The model under review builds one solid part; all positions refer to its coordinate system, in mm. A direction names the side the tool comes from. Coordinates: 2 decimals unless noted, no trailing zeros. Order: outer loops, then holes, each group sorted by start corner. A loop starts at its lowest first (then second) coordinate and runs counter-clockwise, first axis right, second up. Notation, with made-up numbers: (36, 5.5) -> (40, 5.5) arc R23 ccw to (40, 28.5) -> close; hole circle Ø5 at (18.5, 70). An arc over 180 degrees is marked (long way). Use one line per item in the form item = value.
from build123d import *

# Parameters (mm, degrees)
ESQUISSE1_W      = 112
ESQUISSE1_H      = 112
ESQUISSE1_R      = 1.5
EXTRUSION1_DEPTH = 3
ESQUISSE2_W      = 50.8
ESQUISSE2_H      = 25.4
EXTRUSION2_DEPTH = 10
CONG_1_R         = 2
ESQUISSE3_W      = 10
ESQUISSE3_H      = 10
EXTRUSION3_DEPTH = 10
ESQUISSE4_W      = 30
ESQUISSE4_H      = 10
EXTRUSION4_DEPTH = 25
ESQUISSE6_W      = 25
ESQUISSE6_H      = 5
EXTRUSION6_DEPTH = 10


with BuildPart() as part:
    # Esquisse1 → Extrusion1 (new body)
    with BuildSketch(Plane(origin=(0, 0, 0), x_dir=(1, 0, 0), z_dir=(0, 1, 0))):
        with Locations((56, 56)):
            Rectangle(ESQUISSE1_W, ESQUISSE1_H)
        with Locations((3.55, 108.45)):
            Circle(ESQUISSE1_R, mode=Mode.SUBTRACT)
        with Locations((108.45, 108.45)):
            Circle(ESQUISSE1_R, mode=Mode.SUBTRACT)
        with Locations((108.45, 3.55)):
            Circle(ESQUISSE1_R, mode=Mode.SUBTRACT)
        with Locations((3.55, 3.55)):
            Circle(ESQUISSE1_R, mode=Mode.SUBTRACT)
    extrude(amount=EXTRUSION1_DEPTH)

    # Esquisse2 → Extrusion2 (add)
    with BuildSketch(Plane(origin=(0, 3, 0), x_dir=(1, 0, 0), z_dir=(0, 1, 0))):
        with Locations((76.797974596, 22.38755788)):
            Rectangle(ESQUISSE2_W, ESQUISSE2_H)
    extrude(amount=EXTRUSION2_DEPTH)

    # Congé1
    cong_1_edges = [part.edges().sort_by_distance(p)[0] for p in [
        (51.397974596, 13, -22.38755788),
        (76.797974596, 13, -9.68755788),
        (102.197974596, 13, -22.38755788),
        (76.797974596, 13, -35.08755788),
    ]]
    fillet(cong_1_edges, radius=CONG_1_R)

    # Esquisse3 → Extrusion3 (add)
    with BuildSketch(Plane(origin=(0, 3, 0), x_dir=(1, 0, 0), z_dir=(0, 1, 0))):
        with Locations((110.289997157, 97.226447648)):
            Rectangle(ESQUISSE3_W, ESQUISSE3_H)
        with Locations((110.289997157, 67.226447648)):
            Rectangle(ESQUISSE3_W, ESQUISSE3_H)
        with Locations((110.289997157, 52.226447648)):
            Rectangle(ESQUISSE3_W, ESQUISSE3_H)
        with Locations((110.289997157, 82.226447648)):
            Rectangle(ESQUISSE3_W, ESQUISSE3_H)
    extrude(amount=EXTRUSION3_DEPTH)

    # Esquisse4 → Extrusion4 (add)
    with BuildSketch(Plane(origin=(0, 3, 0), x_dir=(1, 0, 0), z_dir=(0, 1, 0))):
        with Locations((61.461032567, 56.630717004)):
            Rectangle(ESQUISSE4_W, ESQUISSE4_H)
        with Locations((61.461032567, 70.501921666)):
            Rectangle(ESQUISSE4_W, ESQUISSE4_H)
        with Locations((31.569885157, 19.889690111)):
            Rectangle(ESQUISSE4_W, ESQUISSE4_H)
        with Locations((61.461032567, 87.97905365)):
            Rectangle(ESQUISSE4_W, ESQUISSE4_H)
    extrude(amount=EXTRUSION4_DEPTH)

    # Esquisse6 → Extrusion6 (add)
    with BuildSketch(Plane(origin=(0, 3, 0), x_dir=(1, 0, 0), z_dir=(0, 1, 0))):
        with Locations((23.111824989, 78.410936793)):
            Rectangle(ESQUISSE6_W, ESQUISSE6_H)
        with Locations((23.111824989, 57.971644922)):
            Rectangle(ESQUISSE6_W, ESQUISSE6_H)
        with Locations((23.111824989, 68.536691251)):
            Rectangle(ESQUISSE6_W, ESQUISSE6_H)
        with Locations((23.111824989, 44.556380649)):
            Rectangle(ESQUISSE6_W, ESQUISSE6_H)
        with Locations((23.111824989, 88.144121685)):
            Rectangle(ESQUISSE6_W, ESQUISSE6_H)
        with Locations((23.111824989, 99.570034384)):
            Rectangle(ESQUISSE6_W, ESQUISSE6_H)
    extrude(amount=EXTRUSION6_DEPTH)


solid = part.part
Item 1: To check wall thickness, follow L1, parallel to Z at x = 3.55, y = 1.25; L2, parallel to X at y = 1.45, z = -3.55; L3, parallel to Z at x = 108, y = 8. State the ranges of each line that lie inside material, in increasing order. Write a range as from..to.
Results found:
L1 = -112..-109.95, -106.95..-5.05, -2.05..0
L2 = 0..2.05, 5.05..106.95, 109.95..112
L3 = -102.23..-92.23, -87.23..-77.23, -72.23..-62.23, -57.23..-47.23
Item 2: We need section A-A (x = 3.55). Write out the cut boundary in (y, z).
Results found:
outline = (0, -112) -> (3, -112) -> (3, -109.95) -> (0, -109.95) -> close; (0, -106.95) -> (3, -106.95) -> (3, -5.05) -> (0, -5.05) -> close; (0, -2.05) -> (3, -2.05) -> (3, 0) -> (0, 0) -> close
Item 3: We need section B-B (z = -108.45). Write out the cut boundary in (x, y), plus the area to 3 significant figures.
Results found:
outline = (0, 0) -> (2.05, 0) -> (2.05, 3) -> (0, 3) -> close; (5.05, 0) -> (106.95, 0) -> (106.95, 3) -> (5.05, 3) -> close; (109.95, 0) -> (112, 0) -> (112, 3) -> (109.95, 3) -> close
area = 318 mm²
Item 4: Draft analysis for pull direction Z (two halves, no side actions). For faces 1 (the face through (31, 15, -24.89)), 2 (the face through (23, 8, -102.07)), 3 (the face through (35.612, 8, -45)), state which applies: released by +Z, released by -Z, zero draft, split by the parting line, or undercut.
Results found:
face_1 = undercut
face_2 = released by -Z
face_3 = zero draft
Item 5: We need section C-C (y = 17.75). Write out the cut boundary in (x, z), plus the area to 3 significant figures.
Results found:
outline = (16.57, -24.89) -> (46.57, -24.89) -> (46.57, -14.89) -> (16.57, -14.89) -> close; (46.46, -92.98) -> (76.46, -92.98) -> (76.46, -82.98) -> (46.46, -82.98) -> close; (46.46, -75.5) -> (76.46, -75.5) -> (76.46, -65.5) -> (46.46, -65.5) -> close; (46.46, -61.63) -> (76.46, -61.63) -> (76.46, -51.63) -> (46.46, -51.63) -> close
area = 1,200 mm²
Item 6: Tool access review of faces 4 (the face through (35.612, 8, -69)), 5 (the face through (102.198, 7, -22)), 6 (the face through (46.57, 15, -20)): name each direction out of +Z, -Z, +X, -X, +Y, -Y from which nothing blocks a thin tool from reaching the whole face with its end or side.
Results found:
face_4 = -Z, +Y
face_5 = +Z, -Z, +X, +Y
face_6 = +Z, +Y
Item 7: Clearance check with flat-ended pins moving along their axes: pin 1 (5.5 mm diameter, centred on x = 26, z = -58.5, fed in from +Y); pin 2 (12 mm diameter, centred on y = 12, z = -53.5, fed in from -X); pin 3 (3.5 mm diameter, centred on y = 1, z = -59, fed in from +X). State where each tip first meets the part, or that it passes through.
Results found:
pin_1 = 13
pin_2 = 10.61
pin_3 = 112
